from build123d import *

# Parameters (mm, degrees)
F2_DEPTH      = 25
F2_DEPTH_BACK = 25
F3_W          = 56
F3_H          = 8
F4_DEPTH      = 25
F4_DEPTH_BACK = 25
F5_R          = 5
F7_R          = 5


with BuildPart() as f1:
    # F0 (on Top) → F1 (revolve)
    with BuildSketch(Plane.XY):
        with BuildLine():
            Line((0, 0), (-3.5, 0))
            ThreePointArc((-3.5, 0), (-7.0355339059, -1.4644660941), (-8.5, -5))
            Line((-8.5, -5), (-8.5, -35))
            Line((-8.5, -35), (0, -35))
            Line((0, -35), (0, -14.25))
            ThreePointArc((0, -14.25), (-4.25, -10), (0, -5.75))
            Line((0, -5.75), (0, 0))
        make_face()
        with BuildLine():
            Line((0, -14.25), (0, -5.75))
            ThreePointArc((0, -5.75), (-4.25, -10), (0, -14.25))
        make_face()
    revolve(axis=Axis((0, -17.5, 0), (0, -1, 0)))

    # F0 (on Top) → F2 (cut, two sides)
    with BuildSketch(Plane.XY) as f2_sk:
        with BuildLine():
            Line((0, -14.25), (0, -5.75))
            ThreePointArc((0, -5.75), (-4.25, -10), (0, -14.25))
        make_face()
        with BuildLine():
            ThreePointArc((4.25, -10), (3.00520382, -6.99479618), (0, -5.75))
            Line((0, -5.75), (0, -14.25))
            ThreePointArc((0, -14.25), (3.00520382, -13.00520382), (4.25, -10))
        make_face()
    extrude(amount=-F2_DEPTH, mode=Mode.SUBTRACT)
    extrude(f2_sk.sketch, amount=F2_DEPTH_BACK, mode=Mode.SUBTRACT)

    # F3 (on Right) → F4 (cut, two sides)
    with BuildSketch(Plane.YZ) as f4_sk:
        Rectangle(F3_W, F3_H)
    extrude(amount=-F4_DEPTH, mode=Mode.SUBTRACT)
    extrude(f4_sk.sketch, amount=F4_DEPTH_BACK, mode=Mode.SUBTRACT)

    # F6: sweep along a path in F0
    with BuildLine(Plane.XY) as f6_path:
        Line((0, -35), (0, -108.6904958737))
        ThreePointArc((0, -108.6904958737), (-0.1379895247, -109.9698836913), (-0.5456110626, -111.1904241367))
        Line((-0.5456110626, -111.1904241367), (-54.4543889374, -228.8095758633))
        ThreePointArc((-54.4543889374, -228.8095758633), (-54.8620104753, -230.0301163087), (-55, -231.3095041263))
        Line((-55, -231.3095041263), (-55, -340))
    # F5 (on face) → F6 (sweep)
    with BuildSketch(Plane.XZ.offset(35)):
        Circle(F5_R)
    sweep(path=f6_path.line)

    # F7
    f7_edges = [f1.edges().sort_by_distance(p)[0] for p in [
        (-60, -340, 0),
    ]]
    fillet(f7_edges, radius=F7_R)


solid = f1.part
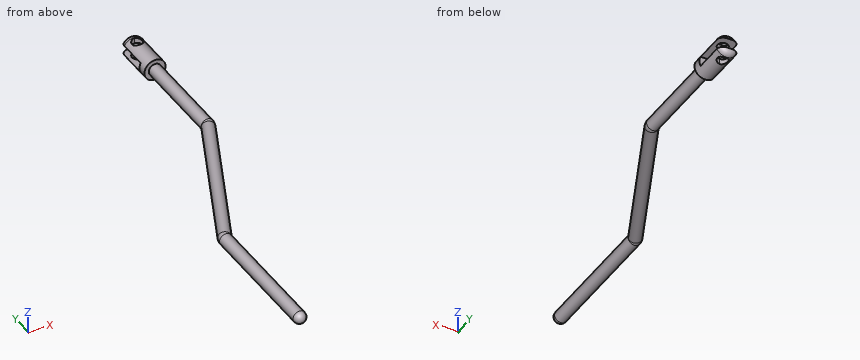
Here's how the part is built. I have some questions about the finished solid (model axes, mm). Coordinates: 2 decimals unless noted, no trailing zeros. Write each loop counter-clockwise with the first axis right and the second up, starting at its lowest first coordinate (ties: lowest second). Pieces come first, ordered by that corner, then holes. Notation, with made-up numbers: (-13.75, -11.75) - (1.25, -11.75) arc R36 cw to (1.25, 23.25) - close; hole circle Ø2 at (60, 8.25). An arc over 180 degrees is marked (long way). Use one line per item in the form item = value.
1) I'm going to push flat-ended pins straight in: P1, Ø2.5, axis at x = -1.5, z = 1, coming from the +Y side; P2, Ø13.5, axis at x = 0, y = -10, coming from the +Z side; P3, Ø3, axis at x = -1.5, z = -3, coming from the +Y side; P4, Ø5, axis at y = -38.5, z = 5.5, coming from the -X side. Where does each tip first touch, or does it pass through?
Solved:
P1 = -28
P2 = 8.5
P3 = -0.03
P4 = -4
2) Suppose I cut it at A-A, the plane z = 0. Write out the boundary of the cut face in (x, y), plus the area to 3 significant figures.
Solved:
outline = (-60, -335) arc R5 ccw to (-50, -335) - (-50, -231.31) arc R1 cw to (-49.91, -230.89) - (4, -113.27) arc R11 ccw to (5, -108.69) - (5, -35) - (8.5, -35) - (8.5, -28) - (-8.5, -28) - (-8.5, -35) - (-5, -35) - (-5, -108.69) arc R1 cw to (-5.09, -109.11) - (-59, -226.73) arc R11 ccw to (-60, -231.31) - close
area = 3,280 mm2
3) I need wall thicknesses on line 1 (X direction, y = -10, z = 6.6); line 2 (Y direction, x = -5, z = -1.25); line 3 (X direction, y = -10, z = 6.2). Which ranges of each line are inside material? Lowest first, please.
Solved:
line_1 = -5.36 to -4.25, 4.25 to 5.36
line_2 = -132.53 to -109.29, -35 to -28
line_3 = -5.81 to -4.25, 4.25 to 5.81
4) Suppose I cut it at B-B, the plane y = -308.5. Write out the boundary of the cut face in (x, z), plus the area to 3 significant figures.
Solved:
outline = circle Ø10 at (-55, 0)
area = 78.5 mm2
